Build history of the part. All positions in model axes, mm. A direction names the side the tool comes from. Round coordinates to 2 decimals unless told otherwise and drop trailing zeros. Write each loop counter-clockwise with the first axis right and the second up, starting at its lowest first coordinate (ties: lowest second). Pieces come first, ordered by that corner, then holes. Notation, with made-up numbers: (56.5, 21) -> (113.5, 21) arc R20 ccw to (113.5, 51) -> close; hole circle Ø3 at (83.5, -5.5). An arc over 180 degrees is marked (long way). Return JSON: item names as keys, results as strings.
Autodesk Inventor part; units mm, degrees
ref_plane "YZ Plane" through (0, 0, 0) normal (1, 0, 0) x (0, 1, 0)
ref_plane "XZ Plane" through (0, 0, 0) normal (0, 1, 0) x (-1, 0, 0)
ref_plane "XY Plane" through (0, 0, 0) normal (0, 0, 1) x (1, 0, 0)
sketch "Sketch1" plane through (0, 0, 0) normal (0, 0, 1) x (1, 0, 0)
  line L0 (0, 0) -> (15, 0)
  line L1 (15, 0) -> (15, 15)
  line L2 (15, 15) -> (0, 15)
  line L3 (0, 15) -> (0, 0)
  dimension "d0" = 15
  dimension "d1" = 15
extrude "Extrusion1" add sketch "Sketch1" along normal blind 10
sketch "Sketch2" plane through (0, 0, 10) normal (0, 0, 1) x (1, 0, 0)
  line L0 (0, 15) -> (7.1003, 15)
  line L1 (15, 15) -> (0, 15)
  line L2 (7.5, 15) -> (7.5, 0)
  line L3 (0, 15) -> (7.9375, 15)
  line L4 (0, 0) -> (0, 7.9375)
  line L5 (0, 7.9375) -> (15, 7.9375)
  circle A0 centre (7.5, 7.9375) radius 4.5
  dimension "d15" = 9
extrude "Extrusion2" add sketch "Sketch2" along normal blind 250
thread "Thread1"
ref_plane "Work Plane1" through (7.5, 7.9375, 260) normal (0, 0, 1) x (1, 0, 0)
sketch "Sketch3" plane through (7.5, 7.9375, 260) normal (0, 0, 1) x (1, 0, 0)
  circle A0 centre (0, 0) radius 5.5
  circle A1 centre (0, 0) radius 4.5
  point P0 (-7.5, -7.9375)
  dimension "d10" = 9
extrude "Extrusion3" add sketch "Sketch3" along normal blind 100 contours A1
thread "Thread2"
properties part number "SA"
Q1. 3-axis set-ups, long thin cutter, end or side, ignore diameter. For faces 1 (the flat face through (15, 7, 5)), 2 (the flat face through (4, 4, 10)): which of +Z, -Z, +X, -X, +Y, -Y reach the whole face in a straight line?
Verdict:
{"face 1": "+Z, -Z, +X, +Y, -Y", "face 2": "+Z"}
Q2. Pin check, flat tips, straight feed: pin 1 Ø2 at (y, z) = (3.5, 168) entering from +X; pin 2 Ø4 at (x, z) = (5.5, 156.5) entering from -Y; pin 3 Ø5 at (x, z) = (3.5, 81) entering from +Y. Stop position of each tip, or through.
Verdict:
{"pin 1": "stops at x = 10.4", "pin 2": "stops at y = 3.44", "pin 3": "stops at y = 12.18"}
Q3. Saw through at A-A on x = 7.5. List the corners of the cut face in (y, z), then the cut area to 3 significant figures.
Verdict:
{"outline": "(0, 0) -> (15, 0) -> (15, 10) -> (12.44, 10) -> (12.44, 360) -> (3.44, 360) -> (3.44, 10) -> (0, 10) -> close", "area": "3,300 mm²"}
Q4. Wall check: L1, parallel to Y at x = 6.75, z = 32; L2, parallel to Z at x = 3.5, y = 14; L3, parallel to Y at x = 4.5, z = 322.5. Give the ranges that are in metal, low to high.
Verdict:
{"L1": "y = 3.5 to 12.37", "L2": "z = 0 to 10", "L3": "y = 4.58 to 11.29"}
Q5. Saw through at B-B on z = 310.5. List the corners of the cut face in (x, y), then the cut area to 3 significant figures.
Verdict:
{"outline": "circle Ø9 at (7.5, 7.94)", "area": "63.6 mm²"}
